Read the model definition and answer for the solid it produces. Units are mm, in the model's axes. A direction names the side the tool comes from. Give positions to 0.01 mm unless a question says otherwise; leave off trailing zeros. Loops run counter-clockwise (first coordinate to the right, second up) from the corner with the lowest first, then second, coordinate; pieces in that order, holes last.
(1) Straight lines are drawn through the part: probe 1 along X at (y, z) = (1, 0); probe 2 along X at (y, z) = (1.1, -2.5); probe 3 along X at (y, z) = (1, -1). For each, find the intervals that lie inside material, in ascending order.
(2) Find section A-A, the plane x = -12.5. Write down the section's boundary in (y, z), then the cut area to 3 significant figures.
(3) Find section C-C, the plane x = 25.65. Write down the section's boundary in (y, z), then the cut area to 3 significant figures.
(4) Find section B-B, the plane z = 0. Write down the section's boundary in (x, y).
(5) Determine the mould class of faces 1 (the face through (0, 3, 8)), 2 (the face through (-15.1, 1, 0)), 3 (the face through (-28.45, 1, 0)) for opening direction X: pulls with the +X half, pulls with the -X half, needs draft (parallel to the pull), parting line crosses it, or undercut.
(6) Which of the six approach directions +Z, -Z, +X, -X, +Y, -Y give full straight-line access (tool end or side, diameter ignored) to faces 4 (the face through (0.21, 0.99, 7.16)), 5 (the face through (-0.2, 2.5, 6.15)), 6 (the face through (27.02, 1.52, -7.5))?
(7) Each of these flat-tipped pins is pushed along its axis until it touches: P1, Ø3, axis at x = 25.65, z = 0, coming from the -Y side; P2, Ø10, axis at x = -5, z = 1.5, coming from the -Y side. Where does it stop, or does it pass through?
Autodesk Inventor part; units mm, degrees
ref_plane "YZ Plane" through (0, 0, 0) normal (1, 0, 0) x (0, 1, 0)
ref_plane "XZ Plane" through (0, 0, 0) normal (0, 1, 0) x (-1, 0, 0)
ref_plane "XY Plane" through (0, 0, 0) normal (0, 0, 1) x (1, 0, 0)
sketch "Skizze1" plane through (0, 0, 0) normal (0, 1, 0) x (-1, 0, 0)
  line L0 (15.1, 6.15) -> (-15.1, 6.15)
  line L1 (-15.1, 6.15) -> (-15.1, -6.15)
  line L2 (-15.1, -6.15) -> (15.1, -6.15)
  line L3 (15.1, -6.15) -> (15.1, 6.15)
  line L4 (15.1, 6.15) -> (-15.1, -6.15) construction
  line L5 (-15.1, 6.15) -> (15.1, -6.15) construction
  line L6 (28.45, 9) -> (-28.45, 9)
  line L7 (-28.45, 9) -> (-28.45, -9)
  line L8 (-28.45, -9) -> (28.45, -9)
  line L9 (28.45, -9) -> (28.45, 9)
  line L10 (28.45, 9) -> (-28.45, -9) construction
  line L11 (-28.45, 9) -> (28.45, -9) construction
  point P0 (0, 0)
  dimension "d0" = 30.2
  dimension "d1" = 12.3
  dimension "d2" = 56.9
  dimension "d3" = 18
extrude "Extrusion1" add sketch "Skizze1" along normal blind 3
chamfer "Fase1" distance 2 angle 45 2 edges at (0, 0, -6.15) (0, 0, 6.15)
sketch "Skizze2" plane through (0, 3, 0) normal (0, 1, 0) x (1, 0, 0)
  line L0 (0, 0) -> (-25.65, 0)
  line L1 (-25.65, 0) -> (25.65, 0)
  dimension "d9" = 25.65
  dimension "d10" = 51.3
hole "Bohrung1" at (25.65, 3, 0) at (-25.65, 3, 0) direction (0, -1, 0) diameter 2.4 end through all countersink diameter 4.4 countersink angle 90
fillet "Rundung1" radius 5 4 edges at (28.45, 1.5, -9) (28.45, 1.5, 9) (-28.45, 1.5, -9) (-28.45, 1.5, 9)
properties part number "Wago2Din_1Way"
Entries:
1. probe 1: x = -28.45 to -26.85, -24.45 to -15.1, 15.1 to 24.45, 26.85 to 28.45
1. probe 2: x = -28.45 to -15.1, 15.1 to 28.45
1. probe 3: x = -28.45 to -26.31, -24.99 to -15.1, 15.1 to 24.99, 26.31 to 28.45
2. outline: (0, -9) - (3, -9) - (3, -6.15) - (2, -6.15) - (0, -8.15) - close; (0, 8.15) - (2, 6.15) - (3, 6.15) - (3, 9) - (0, 9) - close
2. area: 13.1 mm2
3. outline: (0, -8.49) - (3, -8.49) - (3, -2.2) - (2, -1.2) - (0, -1.2) - close; (0, 1.2) - (2, 1.2) - (3, 2.2) - (3, 8.49) - (0, 8.49) - close
3. area: 42.7 mm2
4. outline: (-28.45, 0) - (-26.85, 0) - (-26.85, 2) - (-27.85, 3) - (-28.45, 3) - close; (-24.45, 0) - (-15.1, 0) - (-15.1, 3) - (-23.45, 3) - (-24.45, 2) - close; (15.1, 0) - (24.45, 0) - (24.45, 2) - (23.45, 3) - (15.1, 3) - close; (26.85, 0) - (28.45, 0) - (28.45, 3) - (27.85, 3) - (26.85, 2) - close
5. face 1: needs draft
5. face 2: undercut
5. face 3: pulls with the -X half
6. face 4: -Y
6. face 5: +Y, -Y
6. face 6: -Z, +X, +Y, -Y
7. P1: stops at y = 0
7. P2: stops at y = 1.65
